Check sheet for the modelled part. Datum: model origin and axes. Units: mm. A direction names the side the tool comes from. Round coordinates to 2 decimals unless told otherwise and drop trailing zeros. Order: outer loops, then holes, each group sorted by start corner. A loop starts at its lowest first (then second) coordinate and runs counter-clockwise, first axis right, second up.
```python
from build123d import *

# Parameters (mm, degrees)
F1_DEPTH      = 38.1
F2_DEPTH      = 2.54
F2_DEPTH_BACK = 0.635
F3_DEPTH      = 3.175
F4_START      = -34.925
F4_DEPTH      = 3.175


with BuildPart() as f1:
    # F0 (on Front) → F1 (new body)
    with BuildSketch(Plane.XZ):
        with BuildLine():
            Line((-660.4, 0), (0, 0))
            Line((0, 0), (0, 1676.4))
            ThreePointArc((0, 1676.4), (-44.6369265472, 1784.1630734528), (-152.4, 1828.8))
            Line((-152.4, 1828.8), (-508, 1828.8))
            ThreePointArc((-508, 1828.8), (-615.7630734528, 1784.1630734528), (-660.4, 1676.4))
            Line((-660.4, 1676.4), (-660.4, 0))
        make_face()
        with BuildLine():
            ThreePointArc((-508, 1625.6), (-493.1210244843, 1661.5210244843), (-457.2, 1676.4))
            Line((-457.2, 1676.4), (-203.2, 1676.4))
            ThreePointArc((-203.2, 1676.4), (-167.2789755157, 1661.5210244843), (-152.4, 1625.6))
            Line((-152.4, 1625.6), (-152.4, 1219.2))
            ThreePointArc((-152.4, 1219.2), (-167.2789755157, 1183.2789755157), (-203.2, 1168.4))
            Line((-203.2, 1168.4), (-457.2, 1168.4))
            ThreePointArc((-457.2, 1168.4), (-493.1210244843, 1183.2789755157), (-508, 1219.2))
            Line((-508, 1219.2), (-508, 1625.6))
        make_face(mode=Mode.SUBTRACT)
        with BuildLine():
            Line((-203.2, 1676.4), (-457.2, 1676.4))
            ThreePointArc((-457.2, 1676.4), (-493.1210244843, 1661.5210244843), (-508, 1625.6))
            Line((-508, 1625.6), (-508, 1219.2))
            ThreePointArc((-508, 1219.2), (-493.1210244843, 1183.2789755157), (-457.2, 1168.4))
            Line((-457.2, 1168.4), (-203.2, 1168.4))
            ThreePointArc((-203.2, 1168.4), (-167.2789755157, 1183.2789755157), (-152.4, 1219.2))
            Line((-152.4, 1219.2), (-152.4, 1625.6))
            ThreePointArc((-152.4, 1625.6), (-167.2789755157, 1661.5210244843), (-203.2, 1676.4))
        make_face()
    extrude(amount=-F1_DEPTH)

    # F0 (on Front) → F2 (join, two sides)
    with BuildSketch(Plane.XZ) as f2_sk:
        with BuildLine():
            Line((-676.275, -15.875), (15.875, -15.875))
            Line((15.875, -15.875), (15.875, 1676.4))
            ThreePointArc((15.875, 1676.4), (-33.4116063958, 1795.3883936042), (-152.4, 1844.675))
            Line((-152.4, 1844.675), (-508, 1844.675))
            ThreePointArc((-508, 1844.675), (-626.9883936042, 1795.3883936042), (-676.275, 1676.4))
            Line((-676.275, 1676.4), (-676.275, -15.875))
        make_face()
        with BuildLine():
            Line((0, 1676.4), (0, 0))
            Line((0, 0), (-660.4, 0))
            Line((-660.4, 0), (-660.4, 1676.4))
            ThreePointArc((-660.4, 1676.4), (-615.7630734528, 1784.1630734528), (-508, 1828.8))
            Line((-508, 1828.8), (-152.4, 1828.8))
            ThreePointArc((-152.4, 1828.8), (-44.6369265472, 1784.1630734528), (0, 1676.4))
        make_face(mode=Mode.SUBTRACT)
    extrude(amount=-F2_DEPTH)
    extrude(f2_sk.sketch, amount=F2_DEPTH_BACK)

    # F0 (on Front) → F3 (cut)
    with BuildSketch(Plane.XZ):
        with BuildLine():
            Line((-203.2, 1676.4), (-457.2, 1676.4))
            ThreePointArc((-457.2, 1676.4), (-493.1210244843, 1661.5210244843), (-508, 1625.6))
            Line((-508, 1625.6), (-508, 1219.2))
            ThreePointArc((-508, 1219.2), (-493.1210244843, 1183.2789755157), (-457.2, 1168.4))
            Line((-457.2, 1168.4), (-203.2, 1168.4))
            ThreePointArc((-203.2, 1168.4), (-167.2789755157, 1183.2789755157), (-152.4, 1219.2))
            Line((-152.4, 1219.2), (-152.4, 1625.6))
            ThreePointArc((-152.4, 1625.6), (-167.2789755157, 1661.5210244843), (-203.2, 1676.4))
        make_face()
    extrude(amount=-F3_DEPTH, mode=Mode.SUBTRACT)

    # F0 (on Front) → F4 (cut)
    with BuildSketch(Plane.XZ.offset(F4_START)):
        with BuildLine():
            Line((-203.2, 1676.4), (-457.2, 1676.4))
            ThreePointArc((-457.2, 1676.4), (-493.1210244843, 1661.5210244843), (-508, 1625.6))
            Line((-508, 1625.6), (-508, 1219.2))
            ThreePointArc((-508, 1219.2), (-493.1210244843, 1183.2789755157), (-457.2, 1168.4))
            Line((-457.2, 1168.4), (-203.2, 1168.4))
            ThreePointArc((-203.2, 1168.4), (-167.2789755157, 1183.2789755157), (-152.4, 1219.2))
            Line((-152.4, 1219.2), (-152.4, 1625.6))
            ThreePointArc((-152.4, 1625.6), (-167.2789755157, 1661.5210244843), (-203.2, 1676.4))
        make_face()
    extrude(amount=-F4_DEPTH, mode=Mode.SUBTRACT)


solid = f1.part
```
Item 1: Sectioned sample at D-D (z = 1256). Record the cut outline in (x, y) (3 decimals), and give its area (3 significant figures).
Answer:
outline: (-676.275, -0.635) - (-660.4, -0.635) - (-660.4, 0) - (-508, 0) - (-508, 3.175) - (-152.4, 3.175) - (-152.4, 0) - (0, 0) - (0, -0.635) - (15.875, -0.635) - (15.875, 2.54) - (0, 2.54) - (0, 38.1) - (-152.4, 38.1) - (-152.4, 34.925) - (-508, 34.925) - (-508, 38.1) - (-660.4, 38.1) - (-660.4, 2.54) - (-676.275, 2.54) - close
area: 23,000 mm2
Item 2: Sectioned sample at B-B (x = -377). Record the cut outline in (y, z) (3 decimals), and give its area (3 significant figures).
Answer:
outline: (-0.635, -15.875) - (2.54, -15.875) - (2.54, 0) - (38.1, 0) - (38.1, 1168.4) - (34.925, 1168.4) - (34.925, 1676.4) - (38.1, 1676.4) - (38.1, 1828.8) - (2.54, 1828.8) - (2.54, 1844.675) - (-0.635, 1844.675) - (-0.635, 1828.8) - (0, 1828.8) - (0, 1676.4) - (3.175, 1676.4) - (3.175, 1168.4) - (0, 1168.4) - (0, 0) - (-0.635, 0) - close
area: 66,600 mm2
Item 3: Sectioned sample at A-A (z = 906.5). Record the cut outline in (x, y) (3 decimals), and give its area (3 significant figures).
Answer:
outline: (-676.275, -0.635) - (-660.4, -0.635) - (-660.4, 0) - (0, 0) - (0, -0.635) - (15.875, -0.635) - (15.875, 2.54) - (0, 2.54) - (0, 38.1) - (-660.4, 38.1) - (-660.4, 2.54) - (-676.275, 2.54) - close
area: 25,300 mm2
Item 4: Go/stop test with flat-tipped pins: P1, Ø2, axis at x = -451.5, z = 1500.5, coming from the -Y side (3 decimals); P2, Ø3.5, axis at y = 36.5, z = 1421, coming from the +X side; P3, Ø2, axis at y = 11, z = 930, coming from the -X side. Record where each tip stops, or that it passes through.
Answer:
P1: stops at y = 3.175
P2: stops at x = 0
P3: stops at x = -660.4
Item 5: Release check for a two-part mould opening along X. For faces 6 (the cylindrical face through (-32.11, 0.97, 1794.07)), 7 (the flat face through (-333, 3.175, 1426)) record: released by +X, released by -X, zero draft, split by the parting line, or undercut.
Answer:
face 6: released by +X
face 7: undercut
Item 6: Sectioned sample at C-C (y = 16.5). Record the cut outline in (x, z), and give its area (3 significant figures).
Answer:
outline: (-660.4, 0) - (0, 0) - (0, 1676.4) arc R152.4 ccw to (-152.4, 1828.8) - (-508, 1828.8) arc R152.4 ccw to (-660.4, 1676.4) - close
area: 1,200,000 mm2
Item 7: Access from +Z, -Z, +X, -X, +Y, -Y to the whole of each face (thin tool, end or side, straight path). Record for faces 1 (the flat face through (-333, 34.925, 1426)), 2 (the flat face through (-335, 20, 0)), 3 (the flat face through (-328, 20, 1828.8)), 4 (the flat face through (0, 20, 826)), 5 (the cylindrical face through (-493.514, 1.565, 1183.676)).
Answer:
face 1: +Y
face 2: -Z, +X, -X, +Y
face 3: +Z, +X, -X, +Y
face 4: +Z, -Z, +X, +Y
face 5: -Y
Item 8: Scan lines: line 1 along Y through (x, z) = (-314, 940); line 2 along X through (y, z) = (5, 746.5); line 3 along Z through (x, y) = (-444, 24). Record each from-to range of solid material in increasing order.
Answer:
line 1: y = 0 to 38.1
line 2: x = -660.4 to 0
line 3: z = 0 to 1828.8
